Read the model definition and answer for the solid it produces. Units are mm, in the model's axes. A direction names the side the tool comes from. Round coordinates to 2 decimals unless told otherwise and drop trailing zeros. Order: outer loops, then holes, each group sorted by start corner. A loop starts at its lowest first (then second) coordinate and runs counter-clockwise, first axis right, second up.
Autodesk Fusion 360 part; units mm, degrees
sketch "top" plane through (0, 0, 0) normal (0, 0, 1) x (1, 0, 0)
  line L0 (0, 0) -> (150, 0)
  line L1 (150, 0) -> (150, 33)
  line L2 (150, 33) -> (0, 33)
  line L3 (0, 33) -> (0, 0)
  line L4 (-1, -1) -> (151, -1)
  line L5 (151, -1) -> (151, 34)
  line L6 (151, 34) -> (-1, 34)
  line L7 (-1, 34) -> (-1, -1)
  line L8 (2.5, 2.5) -> (147.5, 2.5)
  line L9 (147.5, 2.5) -> (147.5, 30.5)
  line L10 (147.5, 30.5) -> (2.5, 30.5)
  line L11 (2.5, 30.5) -> (2.5, 2.5)
  line L12 (11, 30.5) -> (11, 34)
  line L13 (-1, 16.5) -> (151, 16.5) construction
  line L14 (75, 34) -> (75, -1) construction
  line L15 (139, 30.5) -> (139, 34)
  line L16 (11, 2.5) -> (11, -1)
  line L17 (139, 2.5) -> (139, -1)
  dimension "d4" = 150
  dimension "d5" = 33
  dimension "d6" = 1
  dimension "d7" = -2.5
  dimension "d8" = 12
extrude "Extrude1" add sketch "top" against normal blind 15 contours L0 L2 L3 L4 L6 L7 L12 L16 | L0 L1 L2 L4 L5 L6 L15 L17 makes body 1 at (-1, 22.3333, -5) makes body 2 at (151, 10.6667, -5)
extrude "Extrude2" add sketch "top" against normal blind 10 contours L0 L4 L16 L17 bodies 1 2
extrude "Extrude3" add sketch "top" against normal blind 1.5 contours L0 L2 L3 L8 L10 L11 L12 L16 | L0 L8 L16 L17 | L0 L1 L2 L8 L9 L10 L15 L17 | L2 L10 L12 L15 bodies 1
extrude "Extrude4" add sketch "top" along normal blind 2.5 contours L0 L2 L3 L8 L10 L11 L12 L16 | L0 L2 L3 L4 L6 L7 L12 L16 | L0 L8 L16 L17 | L0 L4 L16 L17 | L0 L1 L2 L8 L9 L10 L15 L17 | L0 L1 L2 L4 L5 L6 L15 L17 | L2 L10 L12 L15 bodies 1
fillet "Fillet1" radius 3.5 2 edges at (151, 16.5, 2.5) (-1, 16.5, 2.5) on bodies 1
Q1. For a pull along X with two mould halves and no side action, classify faces 1 (the face through (5, 34, -6)), 2 (the face through (145, 33, -8)), 3 (the face through (-1, 17, -8)) as released by +X, released by -X, zero draft, split by the parting line, or undercut.
Outcome:
face 1: zero draft
face 2: undercut
face 3: released by -X
Q2. A cutting plane is placed at A-A, the plane z = -11.5. Give the vertices of the cut face in (x, y).
Outcome:
outline: (-1, -1) - (11, -1) - (11, 0) - (0, 0) - (0, 33) - (11, 33) - (11, 34) - (-1, 34) - close; (139, -1) - (151, -1) - (151, 34) - (139, 34) - (139, 33) - (150, 33) - (150, 0) - (139, 0) - close
Q3. Straight lines are drawn through the part: probe 1 along X at (y, z) = (26, -5.25); probe 2 along X at (y, z) = (17.5, -1); probe 3 along Y at (x, z) = (103.5, -0.5). For each, find the intervals that lie inside material, in ascending order.
Outcome:
probe 1: x = -1 to 0, 150 to 151
probe 2: x = -1 to 2.5, 147.5 to 151
probe 3: y = -1 to 2.5, 30.5 to 33
Q4. A cutting plane is placed at B-B, the plane x = 70. Give the vertices of the cut face in (y, z).
Outcome:
outline: (-1, -10) - (0, -10) - (0, -1.5) - (2.5, -1.5) - (2.5, 2.5) - (-1, 2.5) - close; (30.5, -1.5) - (33, -1.5) - (33, 2.5) - (30.5, 2.5) - close
Q5. For faces 4 (the face through (74, -1, -4)), 5 (the face through (147.5, 16, 1)), 6 (the face through (6, 33, -8)), determine the directions among +Z, -Z, +X, -X, +Y, -Y from which every point of the face is accessible in a straight line to the end or side of a thin tool.
Outcome:
face 4: +Z, -Z, +X, -X, -Y
face 5: +Z, -Z
face 6: -Z
Q6. A cutting plane is placed at D-D, the plane z = 1. Give the vertices of the cut face in (x, y).
Outcome:
outline: (-0.37, -1) - (150.37, -1) - (150.37, 34) - (139, 34) - (139, 33) - (11, 33) - (11, 34) - (-0.37, 34) - close; hole (2.5, 2.5) - (147.5, 2.5) - (147.5, 30.5) - (2.5, 30.5) - close
Q7. Flat-ended cylindrical pins translate along their axes: pin 1 (0.8 mm diameter, centred on x = 105, y = -0.5, fed in from -Z); pin 2 (5 mm diameter, centred on x = 92.5, y = 27.5, fed in from -Z); pin 3 (2 mm diameter, centred on x = 118, z = -4.5, fed in from +Y); pin 4 (2 mm diameter, centred on y = 16.5, z = 0.5, fed in from -X). Find the tip coordinate at first contact, or state that the pin passes through.
Outcome:
pin 1: stops at z = -10
pin 2: passes through
pin 3: stops at y = 0
pin 4: stops at x = -0.96
